Here's how the part is built. I have some questions about the finished solid (model axes, mm). A direction names the side the tool comes from. Coordinates: 2 decimals unless noted, no trailing zeros. Loops run counter-clockwise (first coordinate to the right, second up) from the corner with the lowest first, then second, coordinate; pieces in that order, holes last. Notation, with made-up numbers: (6.5, 11.25) -> (37.5, 11.25) arc R26 cw to (37.5, 38.25) -> close; hole circle Ø10 at (2, -27.5). An arc over 180 degrees is marked (long way). Answer as a JSON object with one key per item and string values. Group by question number.
1) I need wall thicknesses on probe 1 along Z at (x, y) = (-10.5, -43); probe 2 along Y at (x, z) = (0, 8); probe 3 along Y at (x, z) = (0, 10.5). Which ranges of each line are inside material? Lowest first, please. Write a range as [from, to].
2) I want a section at B-B (y = 23.5). Write out the boundary of the cut face in (x, z), then the cut area to 3 significant figures.
3) I'm going to push flat-ended pins straight in: pin 1 (2 mm diameter, centred on x = -31, z = 1.5, fed in from -Y); pin 2 (10 mm diameter, centred on x = -31.5, z = 12, fed in from -Y); pin 3 (12 mm diameter, centred on x = 13.5, z = -7, fed in from +Y); pin 4 (4 mm diameter, centred on x = 56.25, y = 0, fed in from -Z). Where does each tip first touch, or does it pass through?
4) I want a section at A-A (x = 36). Write out the boundary of the cut face in (y, z).
5) I want a section at C-C (z = 11.75). Write out the boundary of the cut face in (x, y), then the cut area to 3 significant figures.
6) If we mould it in two halves opening along X, with no side actions, what happens to faces 1 (the cylindrical face through (-35.97, 35.446, -4.93)), 2 (the cylindrical face through (-44.507, 1.959, 0.838)), 3 (the cylindrical face through (53.653, -0.114, -5.07)), 4 (the cylindrical face through (35.446, 35.97, -4.93))? For each: +X half, -X half, draft (parallel to the pull), parting line (faces both ways), or undercut.
7) Which directions (+Z, -Z, +X, -X, +Y, -Y) give clear straight access to the entire face, cutting with the end or side of a thin tool? Please do faces 5 (the cylindrical face through (35.97, -35.446, -4.93)), 6 (the flat face through (39.4, 16.3, 1.7)), 7 (the flat face through (19, 42, 0)).
```python
from build123d import *

# Parameters (mm, degrees)
SKETCH1_R           = 44.55
BOSS_EXTRUDE1_DEPTH = 15
SKETCH2_R           = 62.5
BOSS_EXTRUDE2_DEPTH = 10
SKETCH3_R           = 40
CUT_EXTRUDE1_DEPTH  = 15
SKETCH4_W           = 4.1
SKETCH4_H           = 2.1
SKETCH7_R           = 2.6
CUT_EXTRUDE4_DEPTH  = 92.855865354
CIRPATTERN1_COUNT   = 4
CUT_EXTRUDE6_DEPTH  = 10


with BuildPart() as part:
    # Sketch1 → Boss-Extrude1 (new body)
    with BuildSketch(Plane.XY):
        Circle(SKETCH1_R)
    extrude(amount=BOSS_EXTRUDE1_DEPTH)

    # Sketch2 → Boss-Extrude2 (add)
    with BuildSketch(Plane(origin=(0, 0, 0), x_dir=(-1, 0, 0), z_dir=(0, 0, -1))):
        Circle(SKETCH2_R)
    extrude(amount=BOSS_EXTRUDE2_DEPTH)

    # Sketch3 → Cut-Extrude1 (cut)
    with BuildSketch(Plane.XY.offset(15)):
        Circle(SKETCH3_R)
    extrude(amount=-CUT_EXTRUDE1_DEPTH, mode=Mode.SUBTRACT)

    # Sketch4 → Cut-Revolve1 (revolve, cut)
    with BuildSketch(Plane(origin=(0, 0, 0), x_dir=(0, 0, -1), z_dir=(1, 0, 0)), mode=Mode.PRIVATE) as cut_revolve1_sk:
        with Locations((-3.75, 43.5)):
            Rectangle(SKETCH4_W, SKETCH4_H)
        with Locations((-11.25, 43.5)):
            Rectangle(SKETCH4_W, SKETCH4_H)
    revolve(cut_revolve1_sk.sketch.rotate(Axis((0, 0, -42.713110189), (0, 0, 1)), 90), axis=Axis((0, 0, -42.713110189), (0, 0, 1)), mode=Mode.SUBTRACT)

    # Sketch7 → Cut-Extrude4 (cut, through all)
    with BuildSketch(Plane(origin=(0, 0, -10), x_dir=(-1, 0, 0), z_dir=(0, 0, -1))):
        with Locations((56.25, 0)):
            Circle(SKETCH7_R)
    cut_extrude4 = extrude(amount=-CUT_EXTRUDE4_DEPTH, mode=Mode.SUBTRACT)

    # CirPattern1: Cut-Extrude4 ×4 about axis
    cirpattern1_axis = Axis((0, 0, 0), (0, 0, 1))
    for i in range(1, CIRPATTERN1_COUNT):
        add(cut_extrude4.rotate(cirpattern1_axis, i * 360 / CIRPATTERN1_COUNT), mode=Mode.SUBTRACT)

    # Sketch10 → Cut-Extrude6 (cut)
    with BuildSketch(Plane.XY):
        with BuildLine():
            ThreePointArc((13.070361778, 48.779254228), (35.70889245, 35.70889245), (48.779254228, 13.070361778))
            add(Edge.make_bspline(
                [(62.4975392, 0.55461157), (62.208727423, 8.100511472), (51.397803822, 7.033582927), (48.779254228, 13.070361778)],
                knots=[0.023286113, 0.023286113, 0.023286113, 0.023286113, 1, 1, 1, 1], degree=3))
            ThreePointArc((62.4975392, 0.55461157), (44.194173824, 44.194173824), (0.55461157, 62.4975392))
            add(Edge.make_bspline(
                [(0.55461157, 62.4975392), (8.100511472, 62.208727423), (7.033582927, 51.397803822), (13.070361778, 48.779254228)],
                knots=[0.023286113, 0.023286113, 0.023286113, 0.023286113, 1, 1, 1, 1], degree=3))
        make_face()
        with BuildLine():
            add(Edge.make_bspline(
                [(62.4975392, -0.55461157), (62.208727423, -8.100511472), (51.397803822, -7.033582927), (48.779254228, -13.070361778)],
                knots=[0.023286113, 0.023286113, 0.023286113, 0.023286113, 1, 1, 1, 1], degree=3))
            ThreePointArc((48.779254228, -13.070361778), (35.70889245, -35.70889245), (13.070361778, -48.779254228))
            add(Edge.make_bspline(
                [(0.55461157, -62.4975392), (8.100511472, -62.208727423), (7.033582927, -51.397803822), (13.070361778, -48.779254228)],
                knots=[0.023286113, 0.023286113, 0.023286113, 0.023286113, 1, 1, 1, 1], degree=3))
            ThreePointArc((0.55461157, -62.4975392), (44.194173824, -44.194173824), (62.4975392, -0.55461157))
        make_face()
        with BuildLine():
            add(Edge.make_bspline(
                [(-0.55461157, -62.4975392), (-8.100511472, -62.208727423), (-7.033582927, -51.397803822), (-13.070361778, -48.779254228)],
                knots=[0.023286113, 0.023286113, 0.023286113, 0.023286113, 1, 1, 1, 1], degree=3))
            ThreePointArc((-13.070361778, -48.779254228), (-35.70889245, -35.70889245), (-48.779254228, -13.070361778))
            add(Edge.make_bspline(
                [(-62.4975392, -0.55461157), (-62.208727423, -8.100511472), (-51.397803822, -7.033582927), (-48.779254228, -13.070361778)],
                knots=[0.023286113, 0.023286113, 0.023286113, 0.023286113, 1, 1, 1, 1], degree=3))
            ThreePointArc((-62.4975392, -0.55461157), (-44.194173824, -44.194173824), (-0.55461157, -62.4975392))
        make_face()
        with BuildLine():
            ThreePointArc((-48.779254228, 13.070361778), (-35.70889245, 35.70889245), (-13.070361778, 48.779254228))
            add(Edge.make_bspline(
                [(-0.55461157, 62.4975392), (-8.100511472, 62.208727423), (-7.033582927, 51.397803822), (-13.070361778, 48.779254228)],
                knots=[0.023286113, 0.023286113, 0.023286113, 0.023286113, 1, 1, 1, 1], degree=3))
            ThreePointArc((-0.55461157, 62.4975392), (-44.194173824, 44.194173824), (-62.4975392, 0.55461157))
            add(Edge.make_bspline(
                [(-62.4975392, 0.55461157), (-62.208727423, 8.100511472), (-51.397803822, 7.033582927), (-48.779254228, 13.070361778)],
                knots=[0.023286113, 0.023286113, 0.023286113, 0.023286113, 1, 1, 1, 1], degree=3))
        make_face()
    extrude(amount=-CUT_EXTRUDE6_DEPTH, mode=Mode.SUBTRACT)


solid = part.part
```
Determined:
{
 "1": {"probe 1": "[-10, 1.7], [5.8, 9.2], [13.3, 15]", "probe 2": "[-44.55, -40], [40, 44.55]", "probe 3": "[-42.45, -40], [40, 42.45]"},
 "2": {"outline": "(-44.7, -10) -> (44.7, -10) -> (44.7, 0) -> (37.85, 0) -> (37.85, 1.7) -> (35.35, 1.7) -> (35.35, 5.8) -> (37.85, 5.8) -> (37.85, 9.2) -> (35.35, 9.2) -> (35.35, 13.3) -> (37.85, 13.3) -> (37.85, 15) -> (32.37, 15) -> (32.37, 0) -> (-32.37, 0) -> (-32.37, 15) -> (-37.85, 15) -> (-37.85, 13.3) -> (-35.35, 13.3) -> (-35.35, 9.2) -> (-37.85, 9.2) -> (-37.85, 5.8) -> (-35.35, 5.8) -> (-35.35, 1.7) -> (-37.85, 1.7) -> (-37.85, 0) -> (-44.7, 0) -> close", "area": "1,020 mm^2"},
 "3": {"pin 1": "y = -32.93", "pin 2": "y = -35.68", "pin 3": "y = 56.25", "pin 4": "through"},
 "4": {"outline": "(-35.42, -10) -> (35.42, -10) -> (35.42, 0) -> (26.24, 0) -> (26.24, 1.7) -> (22.49, 1.7) -> (22.49, 5.8) -> (26.24, 5.8) -> (26.24, 9.2) -> (22.49, 9.2) -> (22.49, 13.3) -> (26.24, 13.3) -> (26.24, 15) -> (17.44, 15) -> (17.44, 0) -> (-17.44, 0) -> (-17.44, 15) -> (-26.24, 15) -> (-26.24, 13.3) -> (-22.49, 13.3) -> (-22.49, 9.2) -> (-26.24, 9.2) -> (-26.24, 5.8) -> (-22.49, 5.8) -> (-22.49, 1.7) -> (-26.24, 1.7) -> (-26.24, 0) -> (-35.42, 0) -> close"},
 "5": {"outline": "circle Ø84.9 at (0, 0); hole circle Ø80 at (0, 0)", "area": "635 mm^2"},
 "6": {"face 1": "-X half", "face 2": "parting line", "face 3": "undercut", "face 4": "+X half"},
 "7": {"face 5": "+Z, -Z, +X, -Y", "face 6": "none", "face 7": "+Z"}
}
